```python
from build123d import *

# Parameters (mm, degrees)
SKETCH1_W           = 211
SKETCH1_H           = 75
BOSS_EXTRUDE1_DEPTH = 4
CUT_EXTRUDE2_REACH  = 114.038
CUT_EXTRUDE3_REACH  = 114.038


with BuildPart() as part:
    # Sketch1 → Boss-Extrude1 (new body)
    with BuildSketch(Plane(origin=(0, 0, 0), x_dir=(1, 0, 0), z_dir=(0, 1, 0))):
        Rectangle(SKETCH1_W, SKETCH1_H)
    extrude(amount=BOSS_EXTRUDE1_DEPTH)

    # Sketch3 → Cut-Extrude2 (cut, up to next)
    with BuildSketch(Plane(origin=(0, 4, 0), x_dir=(1, 0, 0), z_dir=(0, 1, 0)), mode=Mode.PRIVATE) as cut_extrude2_sk1:
        Polygon((-55.5, 37.5), (-55.5, 17.5), (-35.5, 17.5), (-35.5, 21.173298158), (-35.5, 37.5), align=None)
    cut_extrude2_tool1 = extrude(cut_extrude2_sk1.sketch, amount=-CUT_EXTRUDE2_REACH, mode=Mode.PRIVATE) & part.part
    add(cut_extrude2_tool1.solids().sort_by_distance((-45.5, 4, -27.5))[0], mode=Mode.SUBTRACT)

    # Sketch5 → Cut-Extrude3 (cut, up to next)
    with BuildSketch(Plane(origin=(0, 4, 0), x_dir=(1, 0, 0), z_dir=(0, 1, 0)), mode=Mode.PRIVATE) as cut_extrude3_sk1:
        Polygon((44.5, 17.5), (54.5, 17.5), (54.5, 37.5), (34.5, 37.5), (34.5, 17.5), align=None)
    cut_extrude3_tool1 = extrude(cut_extrude3_sk1.sketch, amount=-CUT_EXTRUDE3_REACH, mode=Mode.PRIVATE) & part.part
    add(cut_extrude3_tool1.solids().sort_by_distance((44.5, 4, -27.5))[0], mode=Mode.SUBTRACT)


solid = part.part
```
Input: part model. Units: mm. Frame: model coordinates. A direction names the side the tool comes from. Round coordinates to 2 decimals unless told otherwise and drop trailing zeros. Loops run counter-clockwise (first coordinate to the right, second up) from the corner with the lowest first, then second, coordinate; pieces in that order, holes last. Notation, with made-up numbers: (25.5, 40) - (65.5, 40) arc R17 cw to (65.5, 73) - close; hole circle Ø11 at (80, 52). An arc over 180 degrees is marked (long way). One line per item, written item: value. Start each with the question number.
(1) Section B-B, the plane y = 1.05. Return loops of the section in (x, z).
(2) Section A-A, the plane z = -26.5. Return loops of the section in (x, y), plus the area to 3 significant figures.
(3) Section C-C, the plane x = 41. Return loops of the section in (y, z).
(4) Contact query for flat-ended pins moving along their axis: P1, Ø10, axis at x = 18, z = 14.5, coming from the -Y side; P2, Ø2, axis at x = 46, y = 3, coming from the -Z side. Output: stop coordinate, or through.
(5) Draft query along X for faces 1 (the flat face through (-105.5, 2, 1)), 2 (the flat face through (34.5, 2, -28)), 3 (the flat face through (-1, 2, 37.5)). Return one class per face: +X half, -X half, draft (parallel to the pull), parting line (faces both ways), or undercut.
(6) Access query for faces 4 (the flat face through (54.5, 2, -27)), 5 (the flat face through (-81, 2, -37.5)). Directions: +Z, -Z, +X, -X, +Y, -Y. A direction counts if a zero-diameter tool reaches every point of the face in a straight line with its end or side. Return the directions, or none.
(7) Ray query, line 1 (X direction, y = 2.75, z = -19.5); line 2 (Z direction, x = 48, y = 0.5). Return the intervals inside material, ascending. Write a range as [from, to].
Results below:
1. outline: (-105.5, -37.5) - (-55.5, -37.5) - (-55.5, -17.5) - (-35.5, -17.5) - (-35.5, -37.5) - (34.5, -37.5) - (34.5, -17.5) - (54.5, -17.5) - (54.5, -37.5) - (105.5, -37.5) - (105.5, 37.5) - (-105.5, 37.5) - close
2. outline: (-105.5, 0) - (-55.5, 0) - (-55.5, 4) - (-105.5, 4) - close; (-35.5, 0) - (34.5, 0) - (34.5, 4) - (-35.5, 4) - close; (54.5, 0) - (105.5, 0) - (105.5, 4) - (54.5, 4) - close
2. area: 684 mm^2
3. outline: (0, -17.5) - (4, -17.5) - (4, 37.5) - (0, 37.5) - close
4. P1: y = 0
4. P2: z = -17.5
5. face 1: -X half
5. face 2: undercut
5. face 3: draft
6. face 4: -Z, +Y, -Y
6. face 5: -Z, +X, -X, +Y, -Y
7. line 1: [-105.5, -55.5], [-35.5, 34.5], [54.5, 105.5]
7. line 2: [-17.5, 37.5]
